Work out the finished part from the listing and answer in its coordinate system (mm). Give positions to 0.01 mm unless a question says otherwise; leave off trailing zeros. Order: outer loops, then holes, each group sorted by start corner. A loop starts at its lowest first (then second) coordinate and runs counter-clockwise, first axis right, second up.
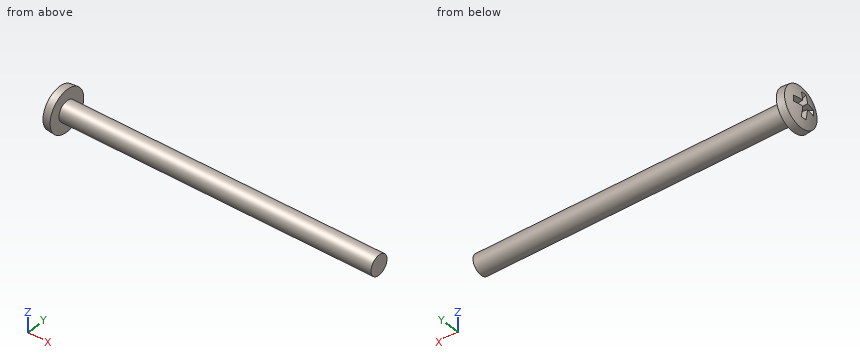
```python
from build123d import *

# Parameters (mm, degrees)
SKETCH3_W         = 0.8636
SKETCH3_H         = 3.9116
SKETCH4_W         = 0.4318
SKETCH4_H         = 0.4318
CIRPATTERN1_COUNT = 2
CIRPATTERN1_ANGLE = 90


with BuildPart() as part:
    # BodySke → Base-Revolve (revolve)
    with BuildSketch(Plane.XY):
        with BuildLine():
            Line((1.7272, 1.4224), (1.7272, 2.9845))
            Line((1.7272, 2.9845), (0.635, 2.888944882))
            ThreePointArc((0.635, 2.888944882), (0.160622478, 1.478954659), (0, 0))
            Line((0, 0), (46.1772, 0))
            Line((46.1772, 0), (46.1772, 1.4224))
            Line((46.1772, 1.4224), (1.7272, 1.4224))
        make_face()
    revolve(axis=Axis((-25.4, 0, 0), (1, 0, 0)))

    # Sketch3 → Cross section 0
    with BuildSketch(Plane(origin=(0, 0, 0), x_dir=(0, 0, -1), z_dir=(1, 0, 0))):
        Rectangle(SKETCH3_W, SKETCH3_H)
    # Sketch4 → Cross section 1
    with BuildSketch(Plane(origin=(2.1844, 0, 0), x_dir=(0, 0, -1), z_dir=(1, 0, 0))):
        Rectangle(SKETCH4_W, SKETCH4_H)
    cross = loft(mode=Mode.SUBTRACT)

    # CirPattern1: Cross ×2 about axis
    cirpattern1_axis = Axis((0, 0, 0), (1, 0, 0))
    for i in range(1, CIRPATTERN1_COUNT):
        add(cross.rotate(cirpattern1_axis, i * CIRPATTERN1_ANGLE / (CIRPATTERN1_COUNT - 1)), mode=Mode.SUBTRACT)


solid = part.part
```
1. Given P1, Ø2, axis at y = -2.5, z = 0.5, coming from the +X side; P2, Ø1.5, axis at y = -0.5, z = -1.5, coming from the +X side; P3, Ø2, axis at x = 8, y = 1, coming from the +Z side; P4, Ø2, axis at x = 10.5, z = 2, coming from the +Y side, each flat-ended and moving along its own axis, determine where each tip first touches the part or whether it passes through.
Findings below:
P1: stops at x = 1.73
P2: stops at x = 46.18
P3: stops at z = 1.42
P4: stops at y = 1.01
2. Straight lines are drawn through the part: probe 1 along X at (y, z) = (-2.25, -0.6); probe 2 along X at (y, z) = (-1.5, 1); probe 3 along Z at (x, y) = (13, -0.15). For each, find the intervals that lie inside material, in ascending order.
Findings below:
probe 1: x = 0.41 to 1.73
probe 2: x = 0.24 to 1.73
probe 3: z = -1.41 to 1.41
3. The part is cut by section A-A (x = 16). Write down the section's boundary in (y, z).
Findings below:
outline: circle Ø2.84 at (0, 0)
